Verification items for the finished model (mm, model axes). Face numbers are marked on the shaded views. A direction names the side the tool comes from. Give positions to 0.01 mm unless a question says otherwise; leave off trailing zeros. Write each loop counter-clockwise with the first axis right and the second up, starting at its lowest first coordinate (ties: lowest second). Pieces come first, ordered by that corner, then holes.
from build123d import *

# Parameters (mm, degrees)
F1_DEPTH = 65
F2_DEPTH = 125


with BuildPart() as f1:
    # F0 (on Top) → F1 (new body)
    with BuildSketch(Plane.XY):
        with BuildLine():
            Line((50, 0), (25, 0))
            ThreePointArc((25, 0), (-17.6776695297, -17.6776695297), (0, 25))
            Line((0, 25), (0, 50))
            ThreePointArc((0, 50), (-35.3553390593, -35.3553390593), (50, 0))
        make_face()
        with BuildLine():
            ThreePointArc((0, 25), (17.6776695297, 17.6776695297), (25, 0))
            Line((25, 0), (50, 0))
            ThreePointArc((50, 0), (35.3553390593, 35.3553390593), (0, 50))
            Line((0, 50), (0, 25))
        make_face()
        with BuildLine():
            ThreePointArc((0, 50), (35.3553390593, 35.3553390593), (50, 0))
            Line((50, 0), (50, 50))
            Line((50, 50), (0, 50))
        make_face()
    extrude(amount=F1_DEPTH)

    # F0 (on Top) → F2 (join)
    with BuildSketch(Plane.XY):
        with BuildLine():
            ThreePointArc((0, 25), (17.6776695297, 17.6776695297), (25, 0))
            Line((25, 0), (50, 0))
            ThreePointArc((50, 0), (35.3553390593, 35.3553390593), (0, 50))
            Line((0, 50), (0, 25))
        make_face()
        with BuildLine():
            ThreePointArc((0, 50), (35.3553390593, 35.3553390593), (50, 0))
            Line((50, 0), (50, 50))
            Line((50, 50), (0, 50))
        make_face()
    extrude(amount=-F2_DEPTH)


solid = f1.part
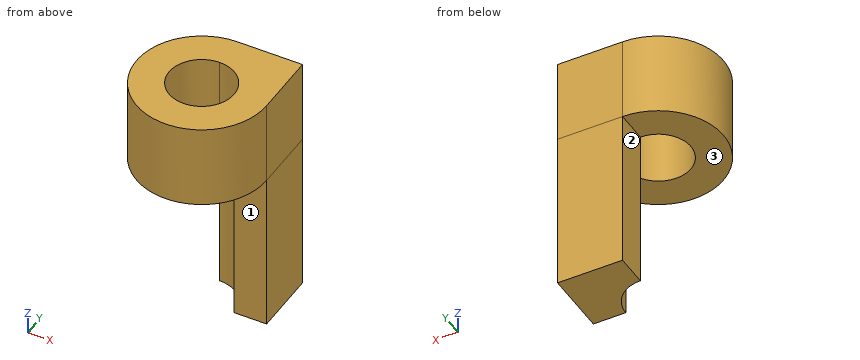
Item 1: Scan lines: line 1 along Y through (x, z) = (0, 37); line 2 along Y through (x, z) = (38.5, -16); line 3 along Z through (x, y) = (39, -27.5). Record each from-to range of solid material in increasing order.
Answer key:
line 1: y = -50 to -25, 25 to 50
line 2: y = 0 to 50
line 3: z = 0 to 65
Item 2: Set-up check for the marked faces 1, 2 and 3: record each of +Z, -Z, +X, -X, +Y, -Y from which the full face is reachable in a straight line by a thin tool's end or side.
Answer key:
face 1: -Z, +X, -X, -Y
face 2: -Z, -X, +Y, -Y
face 3: -Z, -X, -Y
Item 3: Sectioned sample at A-A on x = 21. Record the cut outline in (y, z).
Answer key:
outline: (-45.38, 0) - (-13.56, 0) - (-13.56, 65) - (-45.38, 65) - close; (13.56, -125) - (50, -125) - (50, 65) - (13.56, 65) - close
Item 4: Sectioned sample at B-B on y = 23. Record the cut outline in (x, z).
Answer key:
outline: (-44.4, 0) - (-9.8, 0) - (-9.8, 65) - (-44.4, 65) - close; (9.8, -125) - (50, -125) - (50, 65) - (9.8, 65) - close
Item 5: Sectioned sample at D-D on z = -83.5. Record the cut outline in (x, y), then the cut area to 3 significant figures.
Answer key:
outline: (0, 25) arc R25 cw to (25, 0) - (50, 0) - (50, 50) - (0, 50) - close
area: 2,010 mm2
Item 6: Depth check by flat-ended pin: pin 1 (12.5 mm diameter, centred on y = 34.5, z = -53, fed in from -X); pin 2 (20 mm diameter, centred on x = 41, z = -76, fed in from -Y); pin 3 (1.5 mm diameter, centred on y = 12.5, z = -92.5, fed in from -X). Enter the tip coordinate at first touch or a pass-through.
Answer key:
pin 1: stops at x = 0
pin 2: stops at y = 0
pin 3: stops at x = 21.2
Item 7: Sectioned sample at C-C on z = 36. Record the cut outline in (x, y).
Answer key:
outline: (0, 50) arc R50 ccw (long way) to (50, 0) - (50, 50) - close; hole circle Ø50 at (0, 0)
